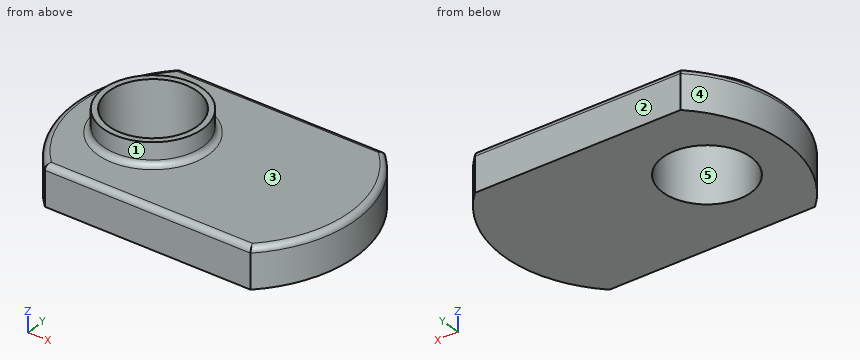
```python
from build123d import *

# Parameters (mm, degrees)
SKETCH1_W                          = 25.4
SKETCH1_H                          = 16.2052
BASE_EXTRUDE_DEPTH                 = 3.6322
SKETCH2_R                          = 4.4958
BOSS_EXTRUDE1_DEPTH                = 2.032
F_5_16_18_TAPPED_HOLE1_D           = 6.5278
F_5_16_18_TAPPED_HOLE1_CBORE_D     = 7.9375
F_5_16_18_TAPPED_HOLE1_CBORE_DEPTH = 15.875
CUT_EXTRUDE1_DEPTH                 = 3.032
CUT_EXTRUDE1_DEPTH_BACK            = 4.6322
CUT_EXTRUDE2_DEPTH                 = 3.032
CUT_EXTRUDE2_DEPTH_BACK            = 4.6322
FILLET1_R                          = 0.508


with BuildPart() as part:
    # Sketch1 → Base-Extrude (new body)
    with BuildSketch(Plane.XY):
        with Locations((12.7, 8.1026)):
            Rectangle(SKETCH1_W, SKETCH1_H)
    extrude(amount=-BASE_EXTRUDE_DEPTH)

    # Sketch2 → Boss-Extrude1 (add)
    with BuildSketch(Plane.XY):
        with Locations((7.112, 8.1026)):
            Circle(SKETCH2_R)
    extrude(amount=BOSS_EXTRUDE1_DEPTH)

    # 5/16-18 Tapped Hole1 (through all)
    with Locations(Plane(origin=(7.112, 8.1026, 2.032), x_dir=(1, 0, 0), z_dir=(0, 0, 1))):
        with Locations((0, 0)):
            CounterBoreHole(F_5_16_18_TAPPED_HOLE1_D / 2, F_5_16_18_TAPPED_HOLE1_CBORE_D / 2, F_5_16_18_TAPPED_HOLE1_CBORE_DEPTH)

    # Sketch4 → Cut-Extrude1 (cut, two sides)
    with BuildSketch(Plane.XY) as cut_extrude1_sk:
        with BuildLine():
            Line((-24.402199862, 61.181765932), (21.971, 16.2052))
            ThreePointArc((21.971, 16.2052), (25.4, 8.1026), (21.971, 0))
            Line((21.971, 0), (-24.402199862, -44.976565932))
            Line((-24.402199862, -44.976565932), (104.800975772, -44.976565932))
            Line((104.800975772, -44.976565932), (104.800975772, 61.181765932))
            Line((104.800975772, 61.181765932), (-24.402199862, 61.181765932))
        make_face()
    extrude(amount=CUT_EXTRUDE1_DEPTH, mode=Mode.SUBTRACT)
    extrude(cut_extrude1_sk.sketch, amount=-CUT_EXTRUDE1_DEPTH_BACK, mode=Mode.SUBTRACT)

    # Sketch6 → Cut-Extrude2 (cut, two sides)
    with BuildSketch(Plane.XY) as cut_extrude2_sk:
        with BuildLine():
            Line((49.802199862, 61.181765932), (3.429, 16.2052))
            ThreePointArc((3.429, 16.2052), (0, 8.1026), (3.429, 0))
            Line((3.429, 0), (49.802199862, -44.976565932))
            Line((49.802199862, -44.976565932), (-79.400975772, -44.976565932))
            Line((-79.400975772, -44.976565932), (-79.400975772, 61.181765932))
            Line((-79.400975772, 61.181765932), (49.802199862, 61.181765932))
        make_face()
    extrude(amount=CUT_EXTRUDE2_DEPTH, mode=Mode.SUBTRACT)
    extrude(cut_extrude2_sk.sketch, amount=-CUT_EXTRUDE2_DEPTH_BACK, mode=Mode.SUBTRACT)

    # Fillet1
    fillet1_edges = [part.edges().sort_by_distance(p)[0] for p in [
        (12.7, 0, 0),
        (0, 8.1026, 0),
        (12.7, 16.2052, 0),
        (2.6162, 8.1026, 0),
        (25.4, 8.1026, 0),
    ]]
    fillet(fillet1_edges, radius=FILLET1_R)


solid = part.part
```
The listing builds one solid part. Answer for the finished solid, in the listing's coordinates (mm). Face numbers are marked on the shaded views. A direction names the side the tool comes from. Coordinates: 2 decimals unless noted, no trailing zeros. Loops run counter-clockwise (first coordinate to the right, second up) from the corner with the lowest first, then second, coordinate; pieces in that order, holes last. Notation, with made-up numbers: (69.5, -34.5) - (127.5, -34.5) arc R5 cw to (127.5, -29.5) - close; hole circle Ø6 at (-32, 81). An arc over 180 degrees is marked (long way). Use a Markdown table: item, result. Add a question column.
1) For the marked faces 1 and 2, determine the directions among +Z, -Z, +X, -X, +Y, -Y from which every point of the face is accessible in a straight line to the end or side of a thin tool.
2) The mould has two halves that part along X. Classify the marked faces 3, 4 and 5: released by +X, released by -X, zero draft, split by the parting line, or undercut.
3) Find the intervals of material crossed by line 1 (Z direction, x = 17, y = 9.75); line 2 (X direction, y = 11, z = 0.25); line 3 (Y direction, x = 6, z = -0.6), in increasing order.
4) The part is cut by section A-A, the plane x = 18.5. Give the vertices of the cut face in (y, z), and give its area (3 significant figures).
5) The part is cut by section C-C, the plane z = 1.1. Give the vertices of the cut face in (x, y).
6) The part is cut by section B-B, the plane z = -2.45. Give the vertices of the cut face in (x, y), and give its area (3 significant figures).
Here are the results:
| question | item | result |
|---|---|---|
| 1 | face 1 | +Z |
| 1 | face 2 | +Z, -Z, +X, -X, +Y |
| 2 | face 3 | zero draft |
| 2 | face 4 | released by -X |
| 2 | face 5 | undercut |
| 3 | line 1 | z = -3.63 to 0 |
| 3 | line 2 | x = 3.58 to 4.4, 9.82 to 10.64 |
| 3 | line 3 | y = 0 to 4.29, 11.91 to 16.21 |
| 4 | outline | (0, -3.63) - (16.21, -3.63) - (16.21, -0.51) arc R0.51 ccw to (15.7, 0) - (0.51, 0) arc R0.51 ccw to (0, -0.51) - close |
| 4 | area | 58.7 mm^2 |
| 5 | outline | circle Ø8.99 at (7.11, 8.1); hole circle Ø7.94 at (7.11, 8.1) |
| 6 | outline | (3.43, 0) - (21.97, 0) arc R11.29 ccw to (21.97, 16.21) - (3.43, 16.21) arc R11.29 ccw to start; hole circle Ø7.94 at (7.11, 8.1) |
| 6 | area | 328 mm^2 |
